For this review, take the finished solid that the model builds, in its own axes (mm). A direction names the side the tool comes from. Give positions to 0.01 mm unless a question says otherwise; leave off trailing zeros. Order: outer loops, then holes, each group sorted by start corner. A loop starts at its lowest first (then second) coordinate and runs counter-clockwise, first axis right, second up. Notation, with made-up numbers: (21.5, -15.5) - (65.5, -15.5) arc R34 cw to (65.5, 14.5) - close; hole circle Ø5 at (60.25, -36.5). An arc over 180 degrees is marked (long way). Answer as a JSON object with one key per item and string values. Group by question number.
from build123d import *

# Parameters (mm, degrees)
SKETCH_1_W          = 3.4775
SKETCH_1_H          = 50
CHAMFER_1_SIZE      = 1
SKETCH_2_OUTSIDE_W  = 34.58
SKETCH_2_OUTSIDE_H  = 34.58
SKETCH_2_OUTSIDE_R  = 9.5
CUT_EXTRUDE_1_DEPTH = 3


with BuildPart() as part:
    # Эскиз1 → Повернуть1 (revolve)
    with BuildSketch(Plane.XY, mode=Mode.PRIVATE) as revolve_1_sk:
        with Locations((8.73875, 25)):
            Rectangle(SKETCH_1_W, SKETCH_1_H)
    revolve(revolve_1_sk.sketch.rotate(Axis((0, 0, 0), (0, 1, 0)), 90), axis=Axis((0, 0, 0), (0, 1, 0)))

    # Фаска1
    chamfer_1_edges = [part.edges().sort_by_distance(p)[0] for p in [
        (0, 0, 10.4775),
    ]]
    chamfer(chamfer_1_edges, length=CHAMFER_1_SIZE)

    # Эскиз2 outside → Вытянуть1 (cut)
    with BuildSketch(Plane(origin=(0, 50, 0), x_dir=(1, 0, 0), z_dir=(0, 1, 0))):
        Rectangle(SKETCH_2_OUTSIDE_W, SKETCH_2_OUTSIDE_H)
        with Locations(Location((0, 0, 0), (0, 0, 270))):
            Circle(SKETCH_2_OUTSIDE_R, mode=Mode.SUBTRACT)
    extrude(amount=-CUT_EXTRUDE_1_DEPTH, mode=Mode.SUBTRACT)


solid = part.part
1) For pin 1 (8.5 mm diameter, centred on x = 0, z = 0, fed in from -Y); pin 2 (12 mm diameter, centred on x = 7, y = 22.5, fed in from -Z); pin 3 (5 mm diameter, centred on y = 32.5, z = 8, fed in from -X); pin 4 (10 mm diameter, centred on x = 7, y = 11, fed in from +Z), all flat-tipped, find the tip position at first contact; note any pin that passes through.
2) Consider section C-C (y = 15). Give the boundary of the cut face in (x, z) (1 decimal), plus the area to 3 significant figures.
3) Consider section A-A (z = 0). Give the boundary of the cut face in (x, y).
4) For line 1 (X direction, y = 38.5, z = 0); line 2 (X direction, y = 17, z = 4); line 3 (Z direction, x = -0.5, y = 11.5), list the stretches that pass through material, from the lowest coordinate up.
5) Mouldability with a two-part tool opening along X and no side actions: class faces 3 (the face through (-10.39, 24.32, 1.36)), 4 (the face through (6.21, 25.35, -3.23)), 5 (the face through (6, 0, -4)) as released by +X, released by -X, zero draft, split by the parting line, or undercut.
6) For faces 1 (the face through (6, 50, -4)), 2 (the face through (4.6, 47, 8.5)), list the 3-axis set-ups (+Z, -Z, +X, -X, +Y, -Y) from which the entire face can be reached by the end or side of a thin tool; tool diameter is ignored.
7) Consider section B-B (x = 0). Give the boundary of the cut face in (y, z), plus the area to 3 significant figures.
Result set:
{
 "1": {"pin 1": "passes through", "pin 2": "stops at z = -10.43", "pin 3": "stops at x = -8.92", "pin 4": "stops at z = 10.28"},
 "2": {"outline": "circle Ø21 at (0, 0); hole circle Ø14 at (0, 0)", "area": "191 mm2"},
 "3": {"outline": "(-10.48, 1) - (-9.48, 0) - (-7, 0) - (-7, 50) - (-9.5, 50) - (-9.5, 47) - (-10.48, 47) - close; (7, 0) - (9.48, 0) - (10.48, 1) - (10.48, 47) - (9.5, 47) - (9.5, 50) - (7, 50) - close"},
 "4": {"line 1": "x = -10.48 to -7, 7 to 10.48", "line 2": "x = -9.68 to -5.74, 5.74 to 9.68", "line 3": "z = -10.47 to -6.98, 6.98 to 10.47"},
 "5": {"face 3": "split by the parting line", "face 4": "undercut", "face 5": "zero draft"},
 "6": {"face 1": "+Z, -Z, +X, -X, +Y", "face 2": "+Y"},
 "7": {"outline": "(0, -9.48) - (1, -10.48) - (47, -10.48) - (47, -9.5) - (50, -9.5) - (50, -7) - (0, -7) - close; (0, 7) - (50, 7) - (50, 9.5) - (47, 9.5) - (47, 10.48) - (1, 10.48) - (0, 9.48) - close", "area": "341 mm2"}
}
